Verification items for the finished model (mm, model axes). A direction names the side the tool comes from. Give positions to 0.01 mm unless a question says otherwise; leave off trailing zeros. Order: outer loops, then holes, each group sorted by start corner. A loop starts at its lowest first (then second) coordinate and runs counter-clockwise, first axis right, second up.
(1) Sectioned sample at B-B on x = 15.5. Record the cut outline in (y, z), plus the area to 3 significant figures.
(2) Mould release check, pull along X, two halves, no side actions. Record for faces 5 (the face through (12.32, -7, -29)), 6 (the face through (0.17, -5.01, 0.55)), 7 (the face through (7.613, -5, 24)), 8 (the face through (19, -18.288, -34)): pulls with the +X half, pulls with the -X half, needs draft (parallel to the pull), parting line crosses it, or undercut.
(3) Gauge pin test, flat ends, axial feed: pin 1 (6 mm diameter, centred on x = 12.5, y = -10.5, fed in from -Z); pin 2 (5.5 mm diameter, centred on y = -12.5, z = -24, fed in from +X); pin 3 (3 mm diameter, centred on x = 21, z = -35, fed in from +Y). Record the tip position at first contact, or that the pin passes through.
(4) Sectioned sample at D-D on x = 0. Record the cut outline in (y, z), plus the area to 3 significant figures.
(5) Access from +Z, -Z, +X, -X, +Y, -Y to the whole of each face (thin tool, end or side, straight path). Record for faces 1 (the face through (0.13, -40.68, -33.7)), 2 (the face through (19, -5, -13.709)), 3 (the face through (0, -10.16, -2)), 4 (the face through (-7.613, -5, 23)).
(6) Sectioned sample at C-C on y = -6. Record the cut outline in (x, z).
(7) Scan lines: L1, parallel to Z at x = -19.5, y = -19; L2, parallel to Y at x = -18.5, z = -22; L3, parallel to X at y = -6.5, z = -15.5. Record each from-to range of solid material in increasing order.
(8) Sectioned sample at A-A on z = 30. Record the cut outline in (x, y).
```python
from build123d import *

# Parameters (mm, degrees)
F1_DEPTH = 10.16
F0_W     = 52.324884
F0_H     = 10.78823
F2_DEPTH = 45.212
F4_DEPTH = 25.4
F5_W     = 14.396261
F5_H     = 25.470311
F6_DEPTH = 18.288


with BuildPart() as f1:
    # F0 (on Front) → F1 (new body)
    with BuildSketch(Plane.XZ):
        with BuildLine():
            Line((26.162442, -28.381733), (26.162442, 39.169963))
            Line((26.162442, 39.169963), (7.613408, 39.169963))
            Line((7.613408, 39.169963), (7.613408, 8.162629))
            ThreePointArc((7.613408, 8.162629), (0, 0.54922), (-7.613408, 8.162629))
            Line((-7.613408, 8.162629), (-7.613408, 39.169963))
            Line((-7.613408, 39.169963), (-26.162442, 39.169963))
            Line((-26.162442, 39.169963), (-26.162442, -28.381733))
            Line((-26.162442, -28.381733), (26.162442, -28.381733))
        make_face()
    extrude(amount=F1_DEPTH)

    # F0 (on Front) → F2 (join)
    with BuildSketch(Plane.XZ):
        with Locations((0, -33.775848)):
            Rectangle(F0_W, F0_H)
    extrude(amount=F2_DEPTH)

    # F3 (on face) → F4 (cut)
    with BuildSketch(Plane.XY.offset(-28.381733)):
        with BuildLine():
            ThreePointArc((26.162442, -33.365056), (-0.258226, -40.668626), (-26.162442, -31.703949))
            Line((-26.162442, -31.703949), (-26.162442, -45.212))
            Line((-26.162442, -45.212), (26.162442, -45.212))
            Line((26.162442, -45.212), (26.162442, -33.365056))
        make_face()
    extrude(amount=-F4_DEPTH, mode=Mode.SUBTRACT)

    # F5 (on face) → F6 (cut)
    with BuildSketch(Plane.XZ):
        with Locations((19.51801, -26.443774)):
            Rectangle(F5_W, F5_H)
    extrude(amount=F6_DEPTH, mode=Mode.SUBTRACT)


solid = f1.part
```
Ans:
1. outline: (-38.42, -39.17) - (-18.29, -39.17) - (-18.29, -28.38) - (-38.42, -28.38) - close; (-10.16, -13.71) - (0, -13.71) - (0, 39.17) - (-10.16, 39.17) - close
1. area: 754 mm2
2. face 5: pulls with the +X half
2. face 6: undercut
2. face 7: undercut
2. face 8: needs draft
3. pin 1: stops at z = -39.17
3. pin 2: stops at x = 12.32
3. pin 3: stops at y = -18.29
4. outline: (-40.68, -39.17) - (0, -39.17) - (0, 0.55) - (-10.16, 0.55) - (-10.16, -28.38) - (-40.68, -28.38) - close
4. area: 733 mm2
5. face 1: +Z, -Z, -Y
5. face 2: -Z, +X, +Y, -Y
5. face 3: +Z, +X, -X, -Y
5. face 4: +Z, +Y, -Y
6. outline: (-26.16, -39.17) - (12.32, -39.17) - (12.32, -13.71) - (26.16, -13.71) - (26.16, 39.17) - (7.61, 39.17) - (7.61, 8.16) arc R7.61 cw to (-7.61, 8.16) - (-7.61, 39.17) - (-26.16, 39.17) - close
7. L1: z = -39.17 to -28.38
7. L2: y = -10.16 to 0
7. L3: x = -26.16 to 12.32
8. outline: (-26.16, -10.16) - (-7.61, -10.16) - (-7.61, 0) - (-26.16, 0) - close; (7.61, -10.16) - (26.16, -10.16) - (26.16, 0) - (7.61, 0) - close
